Part model, mm, in its own coordinate system. A direction names the side the tool comes from. Give positions to 0.01 mm unless a question says otherwise; leave off trailing zeros. Write each loop counter-clockwise with the first axis right and the second up, starting at its lowest first coordinate (ties: lowest second). Pieces come first, ordered by that corner, then holes. Notation, with made-up numbers: M 87.5,81 L 116.5,81 A30 ccw 116.5,112 Z; hole C 54,14.25 d3. An arc over 180 degrees is marked long. Use a Markdown table: item, result.
```python
from build123d import *

# Parameters (mm, degrees)
F1_DEPTH = 66
F2_R     = 2


with BuildPart() as f1:
    # F0 (on Top) → F1 (new body)
    with BuildSketch(Plane.XY):
        with BuildLine():
            Line((-4.1758986024, 2.6), (-1.5758986024, 2.6))
            Line((-1.5758986024, 2.6), (-29.9018225579, 49.3335919775))
            ThreePointArc((-29.9018225579, 49.3335919775), (-31.1664206107, 48.9583804101), (-32.452401675, 49.252054818))
            Line((-32.452401675, 49.252054818), (-4.1758986024, 2.6))
        make_face()
        with BuildLine():
            Line((-31.2494952232, 51.5570528805), (-29.9018225579, 49.3335919775))
            ThreePointArc((-29.9018225579, 49.3335919775), (-28.9841090608, 50.2811118415), (-28.6494952232, 51.5570528805))
            ThreePointArc((-28.6494952232, 51.5570528805), (-31.2494952232, 54.1570528805), (-33.8494952232, 51.5570528805))
            Line((-33.8494952232, 51.5570528805), (-31.2494952232, 51.5570528805))
        make_face()
        with BuildLine():
            ThreePointArc((-32.452401675, 49.252054818), (-31.1664206107, 48.9583804101), (-29.9018225579, 49.3335919775))
            Line((-29.9018225579, 49.3335919775), (-31.2494952232, 51.5570528805))
            Line((-31.2494952232, 51.5570528805), (-33.8494952232, 51.5570528805))
            Line((-33.8494952232, 51.5570528805), (-32.452401675, 49.252054818))
        make_face()
        Polygon((-33, 0), (0, 0), (-1.5758986024, 2.6), (-4.1758986024, 2.6), (-33, 2.6), align=None)
    extrude(amount=F1_DEPTH)

    # F2
    f2_edges = [f1.edges().sort_by_distance(p)[0] for p in [
        (-14.950911, 24.666796, 66),
        (-14.950911, 24.666796, 0),
    ]]
    fillet(f2_edges, radius=F2_R)


solid = f1.part
```
1. Cut at A-A, the plane z = 53. Give the cut face in (x, y).
Findings below:
| item | result |
|---|---|
| outline | M -33.85,51.56 L -4.18,2.6 L -33,2.6 L -33,0 L 0,0 L -29.9,49.33 A2.6 ccw long Z |
2. Drop flat-ended pins along their axis: P1, Ø6, axis at x = -8, y = 16, coming from the -Z side; P2, Ø8.5, axis at x = -19, z = 36.5, coming from the +Y side; P3, Ø1, axis at y = 22, z = 19.5, coming from the -X side; P4, Ø10, axis at x = -17, y = 41, coming from the -Z side. Give the stop position or say it passes through.
Findings below:
| item | result |
|---|---|
| P1 | z = 0.05 |
| P2 | y = 38.36 |
| P3 | x = -16.24 |
| P4 | through |
3. Two-plate mould, pull along Y, no slides. Class faces 4 (the flat face through (-19.22, 27.42, 32.54)), 5 (the flat face through (-17, 0, 33)), 6 (the flat face through (-23, 1, 66)): released by +Y, released by -Y, zero draft, split by the parting line, or undercut.
Findings below:
| item | result |
|---|---|
| face 4 | undercut |
| face 5 | released by -Y |
| face 6 | zero draft |
4. Drill centre lines: L1, parallel to Y at x = -29, z = 18.5; L2, parallel to Y at x = -15.5, z = 27; L3, parallel to Y at x = -30.5, z = 8.5. Where is each one in solid material? Low to high.
Findings below:
| item | result |
|---|---|
| L1 | 0 to 2.6, 43.56 to 47.85, 50.25 to 52.86 |
| L2 | 0 to 2.6, 21.28 to 25.57 |
| L3 | 0 to 2.6, 46.03 to 54.05 |
5. Tool access for faces 1 (the flat face through (-33, 1, 33)), 2 (the flat face through (-23, 1, 0)), 3 (the flat face through (-18, 2.6, 33)): list every direction of +Z, -Z, +X, -X, +Y, -Y with a clear straight run to the whole face (end or side of a thin tool).
Findings below:
| item | result |
|---|---|
| face 1 | +Z, -Z, -X, -Y |
| face 2 | -Z, +X, -X, +Y, -Y |
| face 3 | +Z, -Z, -X |
